Here's the drawing with two shaded views (mm, measured from the low corner). I have some questions. A direction names the side the tool comes from. Round coordinates to 2 decimals unless told otherwise and drop trailing zeros. Loops run counter-clockwise (first coordinate to the right, second up) from the corner with the lowest first, then second, coordinate; pieces in that order, holes last.
(1) I want a section at A-A on x = 8. Write out the boundary of the cut face in (y, z), plus the area to 3 significant figures.
(2) Which directions (+Z, -Z, +X, -X, +Y, -Y) give clear straight access to the entire face, cutting with the end or side of a thin tool? Please do the marked faces 1, 2, 3 and 4.
(3) If I drill on line 1 along Z through (x, y) = (6, 1.8); line 2 along Z through (x, y) = (8, 1.5); line 3 along Y through (x, z) = (3, 6), over which ranges is the centre line in solid material (lowest first)?
(4) Will these pins go through, and if not, where does the flat tip stop? pin 1 Ø2.5 at (y, z) = (5.5, 5) entering from -X; pin 2 Ø4 at (x, y) = (9, 3) entering from +Z; pin 3 Ø2.5 at (x, y) = (9.5, 1.5) entering from -Z.
(5) I want a section at D-D on x = 51.5. Write out the boundary of the cut face in (y, z).
(6) I want a section at B-B on z = 11.25. Write out the boundary of the cut face in (x, y).
(7) Thinking about a two-plate mould opening in X: for the marked faces 5, 6 and 7, which applies, released by +X, released by -X, zero draft, split by the parting line, or undercut?
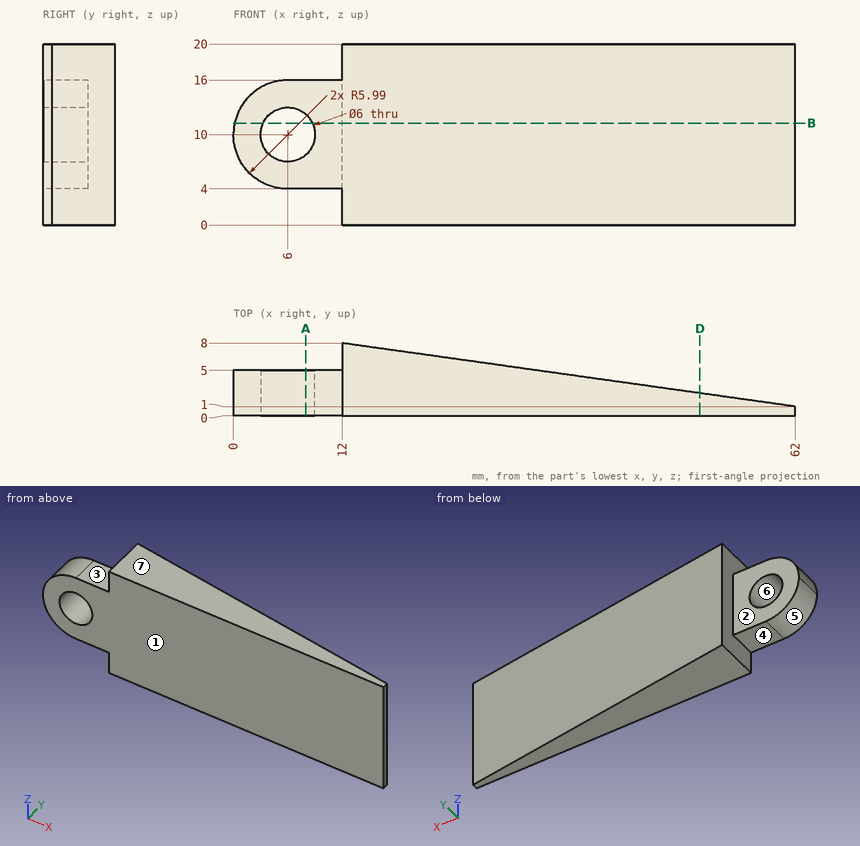
Filled sheet:
1. outline: (0, 4) - (5, 4) - (5, 7.76) - (0, 7.76) - close; (0, 12.24) - (5, 12.24) - (5, 16) - (0, 16) - close
1. area: 37.6 mm2
2. face 1: +Z, -Z, +X, -X, -Y
2. face 2: +Z, -Z, -X, +Y
2. face 3: +Z, -X, +Y, -Y
2. face 4: -Z, -X, +Y, -Y
3. line 1: z = 4 to 7, 13 to 16
3. line 2: z = 4 to 7.76, 12.24 to 16
3. line 3: y = 0 to 5
4. pin 1: stops at x = 1.4
4. pin 2: stops at z = 16
4. pin 3: stops at z = 4
5. outline: (0, 0) - (2.47, 0) - (2.47, 20) - (0, 20) - close
6. outline: (0.13, 0) - (3.27, 0) - (3.27, 5) - (0.13, 5) - close; (8.73, 0) - (62, 0) - (62, 1) - (12, 8) - (12, 5) - (8.73, 5) - close
7. face 5: released by -X
7. face 6: undercut
7. face 7: zero draft
